Verification items for the finished model (mm, model axes). Face numbers are marked on the shaded views. Give positions to 0.01 mm unless a question says otherwise; leave off trailing zeros. Write each loop counter-clockwise with the first axis right and the second up, starting at its lowest first coordinate (ties: lowest second). Pieces come first, ordered by that corner, then holes.
from build123d import *

# Parameters (mm, degrees)
SKETCH1_R           = 25.5
BOSS_EXTRUDE1_DEPTH = 30
SHELL1_T            = -10
SKETCH6_R           = 2.5
BOSS_EXTRUDE2_DEPTH = 1


with BuildPart() as part:
    # Sketch1 → Boss-Extrude1 (new body)
    with BuildSketch(Plane(origin=(0, 0, 0), x_dir=(1, 0, 0), z_dir=(0, 1, 0))):
        with Locations(Location((0, 0, 0), (0, 0, 270))):
            Circle(SKETCH1_R)
    extrude(amount=BOSS_EXTRUDE1_DEPTH)

    # Shell1
    shell1_openings = [part.faces().sort_by_distance(p)[0] for p in [
        (0, 0, 0),
    ]]
    offset(amount=SHELL1_T, openings=shell1_openings, kind=Kind.INTERSECTION)

    # Sweep1: sweep along a path in Sketch5
    with BuildLine(Plane(origin=(0, 0, 0), x_dir=(0, 0, -1), z_dir=(1, 0, 0))) as sweep1_path:
        ThreePointArc((0, 10), (-39.105669761, 22.154641912), (-80, 20))
    # Sketch4 → Sweep1 (sweep)
    with BuildSketch(Plane.XY.offset(80)):
        with BuildLine():
            Line((5, 16), (-5, 16))
            ThreePointArc((-5, 16), (-9, 20), (-5, 24))
            Line((-5, 24), (5, 24))
            ThreePointArc((5, 24), (9, 20), (5, 16))
        make_face()
    sweep(path=sweep1_path.line)

    # Sketch6 → Boss-Extrude2 (add)
    with BuildSketch(Plane(origin=(0, 30, 0), x_dir=(1, 0, 0), z_dir=(0, 1, 0))):
        with Locations(Location((-11.041823898, -12.75, 0), (0, 0, 270))):
            Circle(SKETCH6_R)
        with Locations(Location((11.041823898, -12.75, 0), (0, 0, 90))):
            Circle(SKETCH6_R)
    extrude(amount=BOSS_EXTRUDE2_DEPTH)


solid = part.part
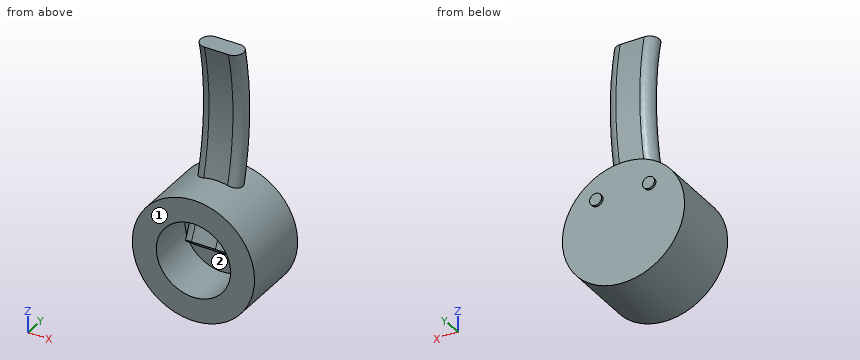
Item 1: Sectioned sample at C-C on x = 16.5. Record the cut outline in (y, z).
Answer key:
outline: (0, -19.44) - (30, -19.44) - (30, 19.44) - (0, 19.44) - close
Item 2: Sectioned sample at A-A on z = -9. Record the cut outline in (x, y), then the cut area to 3 significant figures.
Answer key:
outline: (-23.86, 0) - (-12.62, 0) - (-12.62, 20) - (12.62, 20) - (12.62, 0) - (23.86, 0) - (23.86, 30) - (-23.86, 30) - close
area: 927 mm2
Item 3: Release check for a two-part mould opening along Z. For the marked faces 1 and 2 record: released by +Z, released by -Z, zero draft, split by the parting line, or undercut.
Answer key:
face 1: zero draft
face 2: undercut
Item 4: Scan lines: line 1 along X through (y, z) = (13.5, 0); line 2 along X through (y, z) = (6, 0); line 3 along Z through (x, y) = (-7, 2). Record each from-to range of solid material in increasing order.
Answer key:
line 1: x = -25.5 to -15.5, -7.4 to 7.4, 15.5 to 25.5
line 2: x = -25.5 to -15.5, 15.5 to 25.5
line 3: z = -24.52 to -13.83, 13.83 to 24.52
Item 5: Depth check by flat-ended pin: pin 1 (3 mm diameter, centred on y = 26, z = 19.5, fed in from +X); pin 2 (1.5 mm diameter, centred on y = 17.5, z = -3.5, fed in from -X); pin 3 (1 mm diameter, centred on y = 19.5, z = 61.5, fed in from -X). Enter the tip coordinate at first touch or a pass-through.
Answer key:
pin 1: stops at x = 18.06
pin 2: stops at x = -25.35
pin 3: stops at x = -7.81
Item 6: Sectioned sample at B-B on x = 0. Record the cut outline in (y, z), then the cut area to 3 significant figures.
Answer key:
outline: (0, -25.5) - (30, -25.5) - (30, 25.5) - (23.64, 25.5) arc R120.19 ccw to (24, 80) - (16, 80) arc R112.4 cw to (15.61, 25.5) - (0, 25.5) - (0, 15.5) - (12.53, 15.5) arc R112.4 cw to (6.96, 2.6) - (13.04, -2.6) arc R120.19 ccw to (20, 13.25) - (20, -15.5) - (0, -15.5) - close
area: 1,470 mm2
